Verification items for the finished model (mm, model axes). A direction names the side the tool comes from. Round coordinates to 2 decimals unless told otherwise and drop trailing zeros. Order: outer loops, then holes, each group sorted by start corner. A loop starts at its lowest first (then second) coordinate and runs counter-clockwise, first axis right, second up. Notation, with made-up numbers: M 72,-15 L 86,-15 A24 ccw 86,18 Z; hole C 84.25,-5.75 d3. An arc over 180 degrees is marked long. Use one line per item in the form item = value. Start each with the question number.
Item 1: Release check for a two-part mould opening along Y. For faces 5 (the flat face through (-63, -34, 2)), 6 (the flat face through (56, 40, 2)), 7 (the cylindrical face through (72.581, 21.206, 2.986)), 8 (the flat face through (-74.5, -13.1, 4)) record: +Y half, -Y half, draft (parallel to the pull), parting line (faces both ways), or undercut.
Item 2: Cross-section at A-A on y = 3.5. Enter the section's corners in (x, z), then the cut area to 3 significant figures.
Item 3: Go/stop test with flat-tipped pins: pin 1 Ø0.6 at (x, z) = (42, 3.5) entering from -Y; pin 2 Ø3 at (x, y) = (88.5, -30) entering from +Z; pin 3 Ø8.5 at (x, y) = (83.5, -18) entering from +Z; pin 4 Ø1.5 at (y, z) = (-43, 1) entering from +X. Record where each tip stops, or that it passes through.
Item 4: Cross-section at C-C on y = -44.5. Enter the section's corners in (x, z).
Item 5: Tool access check on faces 1 (the flat face through (77, 16, 2)), 2 (the flat face through (69, -40, 2)), 3 (the flat face through (-44, -5, 2)), 4 (the flat face through (-96, -40, 2)). Record the directions out of +Z, -Z, +X, -X, +Y, -Y that give a thin tool (end or side, any length) a straight path to the whole face; none if there is none.
Item 6: Cross-section at B-B on z = 1. Count the separate pieces of the cut face and the enclosed holes in it, then the cut area to 3 significant figures.
Item 7: Thickness scan on probe 1 along Y at (x, z) = (19.5, 0.6); probe 2 along Y at (x, z) = (-72.5, 0.8); probe 3 along X at (y, z) = (8, 2.6). Record the ranges inside material, lowest first. Write a range as [from, to].
from build123d import *

# Parameters (mm, degrees)
ESQUISSE1_W             = 197
ESQUISSE1_H             = 80
ESQUISSE1_R             = 1.6
BOSS_EXTRU_1_DEPTH      = 2
ESQUISSE2_W             = 110
ESQUISSE2_H             = 45
ENL_V_MAT_EXTRU_1_DEPTH = 2
BOSS_EXTRU_6_DEPTH      = 2
BOSS_EXTRU_2_DEPTH      = 2
ESQUISSE4_W             = 3
ESQUISSE4_H             = 52
BOSS_EXTRU_3_DEPTH      = 2
ESQUISSE5_W             = 3
ESQUISSE5_H             = 74
BOSS_EXTRU_4_DEPTH      = 2
ESQUISSE6_R             = 4.5
ESQUISSE6_R_2           = 1.6
BOSS_EXTRU_5_DEPTH      = 2
ENL_V_MAT_EXTRU_2_DEPTH = 10
ESQUISSE9_R             = 1.6
ENL_V_MAT_EXTRU_3_DEPTH = 2
ESQUISSE10_R            = 4.6
ESQUISSE10_R_2          = 1.6
BOSS_EXTRU_7_DEPTH      = 2
CONG_14_R               = 2


with BuildPart() as part:
    # Esquisse1 → Boss.-Extru.1 (new body)
    with BuildSketch(Plane.XY):
        Rectangle(ESQUISSE1_W, ESQUISSE1_H)
        with Locations((-88.5, -30)):
            Circle(ESQUISSE1_R, mode=Mode.SUBTRACT)
        with Locations((88.5, 30)):
            Circle(ESQUISSE1_R, mode=Mode.SUBTRACT)
        with Locations((88.5, -30)):
            Circle(ESQUISSE1_R, mode=Mode.SUBTRACT)
        with Locations((-88.5, 30)):
            Circle(ESQUISSE1_R, mode=Mode.SUBTRACT)
        with Locations((45, 25)):
            Circle(ESQUISSE1_R, mode=Mode.SUBTRACT)
        with Locations((75, 25)):
            Circle(ESQUISSE1_R, mode=Mode.SUBTRACT)
        with Locations((45, -25)):
            Circle(ESQUISSE1_R, mode=Mode.SUBTRACT)
        with Locations((75, -25)):
            Circle(ESQUISSE1_R, mode=Mode.SUBTRACT)
    extrude(amount=BOSS_EXTRU_1_DEPTH)

    # Esquisse2 → Enlèv. mat.-Extru.1 (cut)
    with BuildSketch(Plane.XY.offset(2)):
        with Locations((-43.5, 17.5)):
            Rectangle(ESQUISSE2_W, ESQUISSE2_H)
    extrude(amount=-ENL_V_MAT_EXTRU_1_DEPTH, mode=Mode.SUBTRACT)

    # Esquisse8 → Boss.-Extru.6 (add)
    with BuildSketch(Plane.XY.offset(2)):
        Polygon((-91.779056191, -40), (-78.5, -63), (26.5, -63), (39.779056191, -40), align=None)
    extrude(amount=-BOSS_EXTRU_6_DEPTH)

    # Esquisse3 → Boss.-Extru.2 (add)
    with BuildSketch(Plane.XY.offset(2)):
        Polygon((98.5, 40), (11.5, 40), (11.5, -5), (-98.5, -5), (-98.5, -40), (-91.779056191, -40), (-78.5, -63), (26.5, -63), (39.779056191, -40), (98.5, -40), align=None)
        Polygon((95.5, 37), (14.5, 37), (14.5, -8), (-95.5, -8), (-95.5, -37), (-90.047005384, -37), (-76.767949192, -60), (24.767949192, -60), (38.047005384, -37), (95.5, -37), align=None, mode=Mode.SUBTRACT)
    extrude(amount=BOSS_EXTRU_2_DEPTH)

    # Esquisse4 → Boss.-Extru.3 (add)
    with BuildSketch(Plane.XY.offset(2)):
        Polygon((14.5, -5), (11.5, -5), (11.5, -60), (14.5, -60), (14.5, -8), (98.5, -8), (98.5, -5), align=None)
        with Locations((-40.5, -34)):
            Rectangle(ESQUISSE4_W, ESQUISSE4_H)
    extrude(amount=BOSS_EXTRU_3_DEPTH)

    # Esquisse5 → Boss.-Extru.4 (add)
    with BuildSketch(Plane.XY.offset(2)):
        with Locations((58, 0)):
            Rectangle(ESQUISSE5_W, ESQUISSE5_H)
    extrude(amount=BOSS_EXTRU_4_DEPTH)

    # Esquisse6 → Boss.-Extru.5 (add)
    with BuildSketch(Plane.XY.offset(2)):
        with Locations(Location((-88.5, -30, 0), (0, 0, 180))):
            Circle(ESQUISSE6_R)
        with Locations((-88.5, -30)):
            Circle(ESQUISSE6_R_2, mode=Mode.SUBTRACT)
        with Locations(Location((88.5, -30, 0), (0, 0, 180))):
            Circle(ESQUISSE6_R)
        with Locations((88.5, -30)):
            Circle(ESQUISSE6_R_2, mode=Mode.SUBTRACT)
        with Locations(Location((75, -25, 0), (0, 0, 180))):
            Circle(ESQUISSE6_R)
        with Locations((75, -25)):
            Circle(ESQUISSE6_R_2, mode=Mode.SUBTRACT)
        with Locations(Location((45, -25, 0), (0, 0, 180))):
            Circle(ESQUISSE6_R)
        with Locations((45, -25)):
            Circle(ESQUISSE6_R_2, mode=Mode.SUBTRACT)
        with Locations(Location((45, 25, 0), (0, 0, 180))):
            Circle(ESQUISSE6_R)
        with Locations((45, 25)):
            Circle(ESQUISSE6_R_2, mode=Mode.SUBTRACT)
        with Locations(Location((75, 25, 0), (0, 0, 180))):
            Circle(ESQUISSE6_R)
        with Locations((75, 25)):
            Circle(ESQUISSE6_R_2, mode=Mode.SUBTRACT)
        with Locations(Location((88.5, 30, 0), (0, 0, 180))):
            Circle(ESQUISSE6_R)
        with Locations((88.5, 30)):
            Circle(ESQUISSE6_R_2, mode=Mode.SUBTRACT)
    extrude(amount=BOSS_EXTRU_5_DEPTH)

    # Esquisse7 → Enlèv. mat.-Extru.2 (cut)
    with BuildSketch(Plane.XY.offset(2)):
        with BuildLine():
            Line((71, -14), (71, -21))
            ThreePointArc((71, -21), (65.5, -26.5), (60, -21))
            Line((60, -21), (60, -14))
            ThreePointArc((60, -14), (65.5, -8.5), (71, -14))
        make_face()
    extrude(amount=-ENL_V_MAT_EXTRU_2_DEPTH, mode=Mode.SUBTRACT)

    # Esquisse9 → Enlèv. mat.-Extru.3 (cut)
    with BuildSketch(Plane(origin=(0, 0, 0), x_dir=(-1, 0, 0), z_dir=(0, 0, -1))):
        with Locations((-19.5, -13)):
            Circle(ESQUISSE9_R)
        with Locations((-19.5, -55)):
            Circle(ESQUISSE9_R)
        with Locations((72.5, -13)):
            Circle(ESQUISSE9_R)
        with Locations((72.5, -55)):
            Circle(ESQUISSE9_R)
    extrude(amount=-ENL_V_MAT_EXTRU_3_DEPTH, mode=Mode.SUBTRACT)

    # Esquisse10 → Boss.-Extru.7 (add)
    with BuildSketch(Plane.XY.offset(2)):
        with Locations(Location((-72.5, -13, 0), (0, 0, 180))):
            Circle(ESQUISSE10_R)
        with Locations(Location((-72.5, -13, 0), (0, 0, 180))):
            Circle(ESQUISSE10_R_2, mode=Mode.SUBTRACT)
        with Locations(Location((-72.5, -55, 0), (0, 0, 180))):
            Circle(ESQUISSE10_R)
        with Locations(Location((-72.5, -55, 0), (0, 0, 180))):
            Circle(ESQUISSE10_R_2, mode=Mode.SUBTRACT)
        with Locations(Location((19.5, -13, 0), (0, 0, 180))):
            Circle(ESQUISSE10_R)
        with Locations(Location((19.5, -13, 0), (0, 0, 180))):
            Circle(ESQUISSE10_R_2, mode=Mode.SUBTRACT)
        with Locations(Location((19.5, -55, 0), (0, 0, 180))):
            Circle(ESQUISSE10_R)
        with Locations(Location((19.5, -55, 0), (0, 0, 180))):
            Circle(ESQUISSE10_R_2, mode=Mode.SUBTRACT)
    extrude(amount=BOSS_EXTRU_7_DEPTH)

    # Congé14
    cong_14_edges = [part.edges().sort_by_distance(p)[0] for p in [
        (11.5, -5, 2),
        (-91.779056191, -40, 2),
        (39.779056191, -40, 2),
    ]]
    fillet(cong_14_edges, radius=CONG_14_R)


solid = part.part
Output values:
q1.face_5 = undercut
q1.face_6 = +Y half
q1.face_7 = undercut
q1.face_8 = draft
q2.outline = M 11.5,0 L 98.5,0 L 98.5,4 L 95.5,4 L 95.5,2 L 59.5,2 L 59.5,4 L 56.5,4 L 56.5,2 L 14.5,2 L 14.5,4 L 11.5,4 Z
q2.area = 192 mm2
q3.pin_1 = -40
q3.pin_2 = through
q3.pin_3 = 2
q3.pin_4 = 38.48
q4.outline = M -89.18,0 L 37.18,0 L 37.18,4 L 33.72,4 L 33.72,2 L 14.5,2 L 14.5,4 L 11.5,4 L 11.5,2 L -39,2 L -39,4 L -42,4 L -42,2 L -85.72,2 L -85.72,4 L -89.18,4 Z
q5.face_1 = +Z
q5.face_2 = +Z, -Z, +X, -Y
q5.face_3 = +Z, -Z, -X, +Y
q5.face_4 = +Z, -Z, -X, -Y
q6.separate_pieces = 1
q6.enclosed_holes = 12
q6.area = 13,300 mm2
q7.probe_1 = [-63, -56.6], [-53.4, -14.6], [-11.4, 40]
q7.probe_2 = [-63, -56.6], [-53.4, -14.6], [-11.4, -5]
q7.probe_3 = [11.5, 14.5], [56.5, 59.5], [95.5, 98.5]
